from build123d import *

# Parameters (mm, degrees)
F0_R      = 80
F0_R_2    = 75
F1_DEPTH  = 180
F2_R      = 80
F2_R_2    = 75
F3_DEPTH  = 220
F4_DEPTH  = 30
F5_DEPTH  = 30
F6_R      = 75
F7_DEPTH  = 250
F8_R      = 75
F9_DEPTH  = 250
F10_R     = 75
F11_DEPTH = 500


with BuildPart() as f1:
    # F0 (on Right) → F1 (new body, symmetric)
    with BuildSketch(Plane.YZ):
        Circle(F0_R)
        Circle(F0_R_2, mode=Mode.SUBTRACT)
    extrude(amount=F1_DEPTH, both=True)

    # F4 (add): a face of the model
    f4_faces = [f1.faces().sort_by_distance(p)[0] for p in [
        (-180, -77.7372583002, 0),
    ]]


with BuildPart() as f3:
    # F2 (on Top) → F3 (new body)
    with BuildSketch(Plane.XY):
        Circle(F2_R)
        Circle(F2_R_2, mode=Mode.SUBTRACT)
    extrude(amount=F3_DEPTH)


with BuildPart() as f1_1:
    add(f1.part)

    add(f3.part)  # F4 merges F3
    extrude(f4_faces, amount=F4_DEPTH)

    # F5 (cut): a face of the model
    f5_faces = [f1_1.faces().sort_by_distance(p)[0] for p in [
        (180, -77.7372583002, 0),
    ]]
    extrude(f5_faces, amount=-F5_DEPTH, mode=Mode.SUBTRACT)

    # F6 (on Right) → F7 (cut, symmetric)
    with BuildSketch(Plane.YZ):
        Circle(F6_R)
    extrude(amount=F7_DEPTH, both=True, mode=Mode.SUBTRACT)

    # F8 (on Right) → F9 (cut, symmetric)
    with BuildSketch(Plane.YZ):
        Circle(F8_R)
    extrude(amount=F9_DEPTH, both=True, mode=Mode.SUBTRACT)

    # F10 (on Top) → F11 (cut)
    with BuildSketch(Plane.XY):
        Circle(F10_R)
    extrude(amount=F11_DEPTH, mode=Mode.SUBTRACT)


with BuildPart() as f12_1:
    # F12: copy of F1
    add(f1_1.part)


solid = f1_1.part
CAD build for the part. Positions are in the model's coordinates, mm. A direction names the side the tool comes from. Round coordinates to 2 decimals unless told otherwise and drop trailing zeros. Loops run counter-clockwise (first coordinate to the right, second up) from the corner with the lowest first, then second, coordinate; pieces in that order, holes last.
(1) Cut at C-C (x = -138). Give the cut face in (y, z), plus the area to 3 significant figures.
(2) Drop flat-ended pins along their axis: pin 1 (1.5 mm diameter, centred on y = 28, z = 106.5, fed in from -X); pin 2 (8 mm diameter, centred on x = 16, z = 56, fed in from +Y); pin 3 (1.5 mm diameter, centred on x = 74, y = 59.5, fed in from -Z). Give the stop position or say it passes through.
(3) Which spindle directions (+Z, -Z, +X, -X, +Y, -Y) get a long thin tool onto all of the face, cutting with end or side? Do faces 1 (the cylindrical face through (-10.41, 79.32, 132.9)), 2 (the flat face through (-210, 23.3, 71.5)). Say none if no direction does.
(4) Cut at D-D (x = -66). Give the cut face in (y, z), plus the area to 3 significant figures.
(5) Cut at B-B (z = -34). Give the cut face in (x, y), plus the area to 3 significant figures.
(6) Cut at A-A (y = 0). Give the cut face in (x, z).
(7) Wall check: line 1 along Z through (x, y) = (-88, 0); line 2 along Z through (x, y) = (122, -3). Give the ranges that are in metal, low to high.
Findings below:
1. outline: circle Ø160 at (0, 0); hole circle Ø150 at (0, 0)
1. area: 2,430 mm2
2. pin 1: stops at x = -75.22
2. pin 2: stops at y = 79.09
2. pin 3: stops at z = -54.3
3. face 1: +Z
3. face 2: +Z, -Z, -X, +Y, -Y
4. outline: (-45.21, 66) arc R80 ccw (long way) to (45.21, 66) - (45.21, 220) - (35.62, 220) - (35.62, 66) arc R75 cw (long way) to (-35.62, 66) - (-35.62, 220) - (-45.21, 220) - close
4. area: 4,960 mm2
5. outline: (-210, -72.42) - (150, -72.42) - (150, -66.85) - (-210, -66.85) - close; (-210, 66.85) - (150, 66.85) - (150, 72.42) - (-210, 72.42) - close
5. area: 4,010 mm2
6. outline: (-210, -80) - (150, -80) - (150, -75) - (-210, -75) - close; (-210, 75) - (-75, 75) - (-75, 220) - (-80, 220) - (-80, 80) - (-210, 80) - close; (75, 75) - (150, 75) - (150, 80) - (80, 80) - (80, 220) - (75, 220) - close
7. line 1: z = -80 to -75, 75 to 80
7. line 2: z = -79.94 to -74.94, 74.94 to 79.94
